Autodesk Inventor part; units mm, degrees
ref_plane "YZ Plane" through (0, 0, 0) normal (1, 0, 0) x (0, 1, 0)
ref_plane "XZ Plane" through (0, 0, 0) normal (0, 1, 0) x (-1, 0, 0)
ref_plane "XY Plane" through (0, 0, 0) normal (0, 0, 1) x (1, 0, 0)
sketch "Sketch1" plane through (0, 0, 0) normal (0, 0, 1) x (1, 0, 0)
  line L0 (-24.746, 21.5893) -> (76.854, 21.5893)
  line L1 (76.854, 21.5893) -> (76.854, -80.0107)
  line L2 (76.854, -80.0107) -> (-24.746, -80.0107)
  line L3 (-24.746, -80.0107) -> (-24.746, 21.5893)
  line L4 (-24.746, 21.5893) -> (76.854, -80.0107)
  line L5 (76.854, 21.5893) -> (-24.746, -80.0107)
  circle A0 centre (26.054, -29.2107) radius 12.7
  point P0 (0, 0)
  dimension "d0" = 101.6
  dimension "d1" = 101.6
  dimension "d2" = 25.4
extrude "Extrusion1" add sketch "Sketch1" along normal blind 8.128 and the other way blind 3.937
sketch "Sketch2" plane through (0, 0, 8.128) normal (0, 0, 1) x (1, 0, 0)
  line L0 (-24.746, 21.5893) -> (76.854, -80.0107)
  line L1 (76.854, 21.5893) -> (-24.746, -80.0107)
  circle A0 centre (26.054, -29.2107) radius 12.7
  point P0 (0, 0)
  dimension "d7" = 25.4
extrude "Extrusion2" cut sketch "Sketch2" against normal blind 8.128
sketch "Sketch3" plane through (-24.746, 21.5893, 8.128) normal (0, 1, 0) x (1, 0, 0)
  line L0 (101.6, 12.065) -> (101.6, 0)
  line L1 (101.6, 12.065) -> (0, 12.065)
  line L2 (0, 0) -> (0, 12.065)
  line L3 (0, 12.065) -> (101.6, 12.065)
  line L4 (101.6, 12.065) -> (101.6, 11.303)
  line L5 (101.6, 11.303) -> (0, 11.303)
  line L6 (0, 11.303) -> (0, 12.065)
  line L7 (101.6, 0) -> (0, 0)
  line L8 (0, 0) -> (0, 0.762)
  line L9 (0, 0.762) -> (101.6, 0.762)
  line L10 (101.6, 0.762) -> (101.6, 0)
  line L11 (0, 0.762) -> (0, 11.303)
  line L12 (101.6, 12.065) -> (101.6, 0.762)
  point P0 (24.746, 8.128)
  dimension "d10" = 0.762
  dimension "d11" = 0.762
extrude "Extrusion3" cut sketch "Sketch3" against normal blind 101.6 contours L0 L9 L2 L5
sketch "Sketch4" plane through (0, 0, 8.128) normal (0, 0, 1) x (1, 0, 0)
  circle A0 centre (26.054, -29.2107) radius 12.7
  circle A1 centre (26.054, -29.2107) radius 19.05
  point P0 (0, 0)
  dimension "d14" = 38.1
extrude "Extrusion4" add sketch "Sketch4" against normal blind 8.128
sketch "Sketch5" plane through (0, 0, 8.128) normal (0, 0, 1) x (1, 0, 0)
  circle A0 centre (26.054, -29.2107) radius 12.7
  point P0 (0, 0)
extrude "Extrusion5" cut sketch "Sketch5" against normal blind 25.4
sketch "Sketch6" plane through (26.054, -29.2107, 0) normal (0, 0, -1) x (-1, 0, 0)
  circle A0 centre (0, 0) radius 12.7
  circle A1 centre (0, 0) radius 19.05
  point P0 (26.054, 29.2107)
extrude "Extrusion6" add sketch "Sketch6" along normal blind 3.556
properties part number "lazysusanbasic"
Could you check a few things on this model? Use its own coordinates, in mm. Give positions to 0.01 mm unless a question says otherwise; leave off trailing zeros. Write each loop counter-clockwise with the first axis right and the second up, starting at its lowest first coordinate (ties: lowest second). Pieces come first, ordered by that corner, then holes. Notation, with made-up numbers: (34.5, 31) - (69.5, 31) arc R23 ccw to (69.5, 70) - close; hole circle Ø11 at (26.25, 82). An arc over 180 degrees is marked (long way). Use CSV: the item, a comma, the result in double quotes. Start each with the question number.
Item 1: I want a section at A-A, the plane x = -16.5. Please give me the cut outline in (y, z) (3 decimals).
Item 2: I want a section at B-B, the plane y = -70.5. Please give me the cut outline in (x, z) (3 decimals), then the cut area to 3 significant figures.
Item 3: If we mould it in two halves opening along Z, with no side actions, what happens to faces 1 (the face through (25, -6, 7.366)), 2 (the face through (14, -17, -3.937)), 3 (the face through (14, -17, 8.128))? For each: pulls with the +Z half, pulls with the -Z half, needs draft (parallel to the pull), parting line crosses it, or undercut.
Item 4: If I drill on line 1 along Z through (x, y) = (71, -58.5) (3 decimals); line 2 along Y through (x, z) = (26.5, 7.25); line 3 along Y through (x, z) = (15.5, 1.25), over which ranges is the centre line in solid material (lowest first)?
Item 5: I want a section at D-D, the plane x = 10. Please give me the cut outline in (y, z) (3 decimals), then the cut area to 3 significant figures.
Item 6: I want a section at C-C, the plane z = -1.5. Please give me the cut outline in (x, y).
Item 7: I'm going to push flat-ended pins straight in: pin 1 (1 mm diameter, centred on x = 47.5, z = 4, fed in from -Y); pin 2 (1 mm diameter, centred on y = -22.5, z = 0.5, fed in from -X); pin 3 (3 mm diameter, centred on y = -33, z = 3, fed in from +X). Where does each tip first touch, or does it pass through?
Findings:
1,outline,"(-80.011, -3.937) - (21.589, -3.937) - (21.589, -3.175) - (-80.011, -3.175) - close; (-80.011, 7.366) - (21.589, 7.366) - (21.589, 8.128) - (-80.011, 8.128) - close"
2,outline,"(-24.746, -3.937) - (76.854, -3.937) - (76.854, -3.175) - (-24.746, -3.175) - close; (-24.746, 7.366) - (76.854, 7.366) - (76.854, 8.128) - (-24.746, 8.128) - close"
2,area,"155 mm2"
3,face 1,"undercut"
3,face 2,"pulls with the -Z half"
3,face 3,"pulls with the +Z half"
4,line 1,"z = -3.937 to -3.175, 7.366 to 8.128"
4,line 2,"y = -48.26 to -41.9, -16.52 to -10.17"
4,line 3,"y = -45.07 to -36.27, -22.15 to -13.35"
5,outline,"(-80.011, -3.937) - (21.589, -3.937) - (21.589, -3.175) - (-18.955, -3.175) - (-18.955, 7.366) - (21.589, 7.366) - (21.589, 8.128) - (-80.011, 8.128) - (-80.011, 7.366) - (-39.466, 7.366) - (-39.466, -3.175) - (-80.011, -3.175) - close"
5,area,"371 mm2"
6,outline,"circle Ø38.1 at (26.05, -29.21); hole circle Ø25.4 at (26.05, -29.21)"
7,pin 1,"passes through"
7,pin 2,"stops at x = 8.04"
7,pin 3,"stops at x = 44.97"
